Build history of the part. All positions in model axes, mm. Face numbers are marked on the shaded views. Round coordinates to 2 decimals unless told otherwise and drop trailing zeros. Write each loop counter-clockwise with the first axis right and the second up, starting at its lowest first coordinate (ties: lowest second). Pieces come first, ordered by that corner, then holes. Notation, with made-up numbers: M -30.5,57 L -22.5,57 A7 ccw -22.5,65 Z; hole C 49,-12 d5. An arc over 180 degrees is marked long. Write item = value, one per line.
from build123d import *

# Parameters (mm, degrees)
SKETCH1_W                 = 20
SKETCH1_H                 = 40
SKETCH1_R                 = 5
BOSS_EXTRUDE1_DEPTH       = 10
FILLET1_R                 = 3
F_3_0MM_DOWEL_HOLE1_D     = 3
F_3_0MM_DOWEL_HOLE1_DEPTH = 5
F_3_0MM_DOWEL_HOLE1_TIP   = 0.901290929


with BuildPart() as part:
    # Sketch1 → Boss-Extrude1 (new body)
    with BuildSketch(Plane(origin=(0, 0, 0), x_dir=(0, 0, -1), z_dir=(1, 0, 0))):
        Rectangle(SKETCH1_W, SKETCH1_H)
        with Locations((0, 11.27)):
            Circle(SKETCH1_R, mode=Mode.SUBTRACT)
    extrude(amount=BOSS_EXTRUDE1_DEPTH)

    # Fillet1
    fillet1_edges = [part.edges().sort_by_distance(p)[0] for p in [
        (5, 20, 10),
        (5, 20, -10),
        (10, 20, 0),
        (0, 20, 0),
    ]]
    fillet(fillet1_edges, radius=FILLET1_R)

    # Ø3.0mm Dowel Hole1
    with Locations(Plane.XZ.offset(20)):
        with Locations((5, 0)):
            Hole(F_3_0MM_DOWEL_HOLE1_D / 2, depth=F_3_0MM_DOWEL_HOLE1_DEPTH)
            with Locations((0, 0, -(F_3_0MM_DOWEL_HOLE1_DEPTH + F_3_0MM_DOWEL_HOLE1_TIP / 2))):  # 118° drill point
                Cone(0, F_3_0MM_DOWEL_HOLE1_D / 2, F_3_0MM_DOWEL_HOLE1_TIP, mode=Mode.SUBTRACT)


solid = part.part
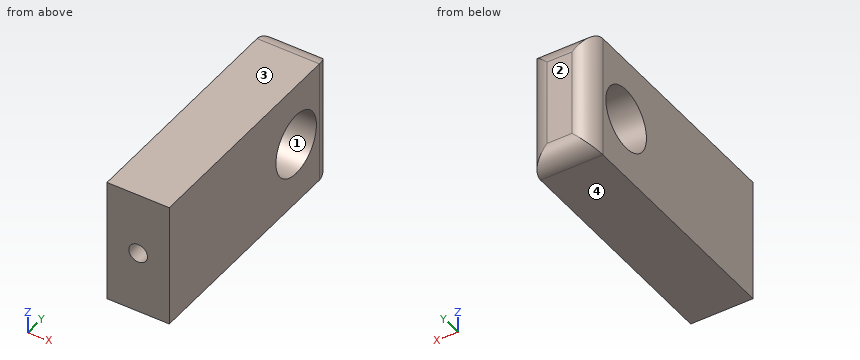
1. Flat gauge pin, fed straight in: pin 1 (6 mm diameter, centred on y = 11.27, z = 0, fed in from -X). Where does the tip first touch, or does it go through?
Responses:
pin_1 = through
2. Band-saw the part on A-A (y = 11.27). List the corners of the cut face in (x, z), plus the area to 3 significant figures.
Responses:
outline = M 0,-10 L 10,-10 L 10,-5 L 0,-5 Z; M 0,5 L 10,5 L 10,10 L 0,10 Z
area = 100 mm²
3. Probe probe 1 along Y at (x, z) = (7, 0); probe 2 along X at (y, z) = (-18.9, 0); probe 3 along Z at (x, y) = (3.25, 12.5). List the from-to ranges inside material, lowest first.
Responses:
probe_1 = -20 to 6.27, 16.27 to 20
probe_2 = 0 to 3.5, 6.5 to 10
probe_3 = -10 to -4.85, 4.85 to 10
4. Band-saw the part on D-D (z = 2.25). List the corners of the cut face in (x, y), plus the area to 3 significant figures.
Responses:
outline = M 0,-20 L 10,-20 L 10,6.8 L 0,6.8 Z; M 0,15.74 L 10,15.74 L 10,17 A3 ccw 7,20 L 3,20 A3 ccw 0,17 Z
area = 307 mm²
5. Band-saw the part on B-B (z = -3). List the corners of the cut face in (x, y), plus the area to 3 significant figures.
Responses:
outline = M 0,-20 L 10,-20 L 10,7.27 L 0,7.27 Z; M 0,15.27 L 10,15.27 L 10,17 A3 ccw 7,20 L 3,20 A3 ccw 0,17 Z
area = 316 mm²
6. Band-saw the part on C-C (x = 2.5). List the corners of the cut face in (y, z).
Responses:
outline = M -20,-10 L 17,-10 A3 ccw 19.96,-7.5 L 19.96,7.5 A3 ccw 17,10 L -20,10 Z; hole C 11.27,0 d10
7. Mould opens along Z. For the marked faces 1, 2, 3 and 4 say: pulls with the +Z half, pulls with the -Z half, needs draft (parallel to the pull), parting line crosses it, or undercut.
Responses:
face_1 = undercut
face_2 = needs draft
face_3 = pulls with the +Z half
face_4 = pulls with the -Z half
